Design review of the part built by this model. Coordinates are the model's own, in mm. A direction names the side the tool comes from. Give positions to 0.01 mm unless a question says otherwise; leave off trailing zeros. Order: outer loops, then holes, each group sorted by start corner. A loop starts at its lowest first (then second) coordinate and runs counter-clockwise, first axis right, second up. Notation, with made-up numbers: (-1.75, 81.25) -> (7.25, 81.25) arc R8 cw to (7.25, 87.25) -> close; hole circle Ø3 at (-8, 67). An arc over 180 degrees is marked (long way). Return JSON: item names as keys, results as strings.
```python
from build123d import *

# Parameters (mm, degrees)
BOSS_EXTRUDE1_DEPTH       = 13
SKETCH2_W                 = 26
SKETCH2_H                 = 9
CUT_EXTRUDE1_DEPTH        = 7
SKETCH3_W                 = 5.460158558
SKETCH3_H                 = 35.727642342
SKETCH3_W_2               = 6.990786849
SKETCH3_H_2               = 37.804269356
CUT_EXTRUDE2_DEPTH        = 56.362442143
M3X0_5_TAPPED_HOLE2_D     = 2.5
M3X0_5_TAPPED_HOLE2_DEPTH = 15
M3X0_5_TAPPED_HOLE2_TIP   = 0.751075774
M3X0_5_TAPPED_HOLE1_D     = 2.5
M3_CLEARANCE_HOLE1_D      = 3.4
CUT_EXTRUDE3_DEPTH        = 58.766772456
FILLET2_R                 = 3
CHAMFER1_SIZE             = 20
CHAMFER1_SIZE_2           = 3
CUT_EXTRUDE4_REACH        = 57.362
FILLET3_R                 = 2
CUT_EXTRUDE5_REACH        = 57.527
FILLET4_R                 = 2
M5X0_8_TAPPED_HOLE1_D     = 4.2
M5X0_8_TAPPED_HOLE1_DEPTH = 11.927025935
FILLET6_R                 = 5
CUT_EXTRUDE6_REACH        = 57.362
SKETCH19_W                = 7
SKETCH19_H                = 16
FILLET7_R                 = 1
CHAMFER2_SIZE             = 1.5
FILLET8_R                 = 0.5
FILLET9_R                 = 1


with BuildPart() as part:
    # Sketch1 → Boss-Extrude1 (new, symmetric)
    with BuildSketch(Plane.XY):
        Polygon((0, 0), (36, 0), (36, 36.17831254), (25.5, 40), (0, 17), align=None)
    extrude(amount=BOSS_EXTRUDE1_DEPTH, both=True)

    # Sketch2 → Cut-Extrude1 (cut)
    with BuildSketch(Plane.ZY):
        with Locations((0, 4.5)):
            Rectangle(SKETCH2_W, SKETCH2_H)
    extrude(amount=-CUT_EXTRUDE1_DEPTH, mode=Mode.SUBTRACT)

    # Sketch3 → Cut-Extrude2 (cut, through all)
    with BuildSketch(Plane.ZY):
        with Locations((10.730079279, 26.863821171)):
            Rectangle(SKETCH3_W, SKETCH3_H)
        with Locations((-11.495393425, 27.902134678)):
            Rectangle(SKETCH3_W_2, SKETCH3_H_2)
    extrude(amount=-CUT_EXTRUDE2_DEPTH, mode=Mode.SUBTRACT)

    # M3x0.5 Tapped Hole2
    with Locations(Plane(origin=(7, 5, -9.5), x_dir=(0, -1, 0), z_dir=(-1, 0, 0))):
        with Locations((0, 0), (0, 19)):
            Hole(M3X0_5_TAPPED_HOLE2_D / 2, depth=M3X0_5_TAPPED_HOLE2_DEPTH)
            with Locations((0, 0, -(M3X0_5_TAPPED_HOLE2_DEPTH + M3X0_5_TAPPED_HOLE2_TIP / 2))):  # 118° drill point
                Cone(0, M3X0_5_TAPPED_HOLE2_D / 2, M3X0_5_TAPPED_HOLE2_TIP, mode=Mode.SUBTRACT)

    # M3x0.5 Tapped Hole1 (through all)
    with Locations(Plane(origin=(3.5, 12.5, 8), x_dir=(1, 0, 0), z_dir=(0, 0, 1))):
        with Locations((0, 0)):
            Hole(M3X0_5_TAPPED_HOLE1_D / 2)

    # M3 Clearance Hole1 (through all)
    with Locations(Plane.XY.offset(13)):
        with Locations((27, 5)):
            Hole(M3_CLEARANCE_HOLE1_D / 2)

    # Sketch13 → Cut-Extrude3 (cut, through all)
    with BuildSketch(Plane.XY.offset(8)):
        Polygon((32, 18.871173631), (32, 26.992415753), (21.34884319, 30.869119792), (7, 17.927025935), (7, 11.927025935), (32, 11.927025935), align=None)
    extrude(amount=-CUT_EXTRUDE3_DEPTH, mode=Mode.SUBTRACT)

    # Fillet2
    fillet2_edges = [part.edges().sort_by_distance(p)[0] for p in [
        (7, 11.927025935, 0),
        (7, 17.927025935, 0),
        (21.34884319, 30.869119792, 0),
        (32, 26.992415753, 0),
        (32, 11.927025935, 0),
    ]]
    fillet(fillet2_edges, radius=FILLET2_R)

    # Chamfer1
    # the kernel refuses this chamfer: 20, 3 mm, written as the material it takes off along each edge
    with BuildSketch(Plane(origin=(84.844019059, 18.400543481, 8), x_dir=(-0.3420145720677014, -0.939677313880462, 0.005707737883485923), z_dir=(-0.9396926207859104, 0.3420201433256634, 0))) as chamfer1_piece_1:
        Polygon((CHAMFER1_SIZE * 0.999983710731, -CHAMFER1_SIZE * 0.00570773788349), (-CHAMFER1_SIZE_2 * 0.00570773788349, -CHAMFER1_SIZE_2 * 0.999983710731), (0, 0), align=None)
    extrude(amount=115.131305413, mode=Mode.SUBTRACT)
    with BuildSketch(Plane(origin=(84.844019059, 18.400543481, -8), x_dir=(0.08410022637244834, 0.23106347292932808, 0.9692970769593502), z_dir=(-0.9396926207859104, 0.3420201433256634, 0))) as chamfer1_piece_2:
        Polygon((CHAMFER1_SIZE_2 * 0.969297076959, -CHAMFER1_SIZE_2 * 0.245892611922), (-CHAMFER1_SIZE * 0.245892611922, -CHAMFER1_SIZE * 0.969297076959), (0, 0), align=None)
    extrude(amount=115.131305413, mode=Mode.SUBTRACT)

    # Sketch14 → Cut-Extrude4 (cut, up to next)
    with BuildSketch(Plane(origin=(36, 0, 0), x_dir=(0, 0, -1), z_dir=(1, 0, 0)), mode=Mode.PRIVATE) as cut_extrude4_sk1:
        Polygon((-3.405017352, 26), (3.405017352, 26), (5.096464069, 14), (-5.096464069, 14), align=None)
    cut_extrude4_tool1 = extrude(cut_extrude4_sk1.sketch, amount=-CUT_EXTRUDE4_REACH, mode=Mode.PRIVATE) & part.part
    add(cut_extrude4_tool1.solids().sort_by_distance((36, 19.602082, 0))[0], mode=Mode.SUBTRACT)

    # Fillet3
    fillet3_edges = [part.edges().sort_by_distance(p)[0] for p in [
        (33.926588844, 14, -5.096464069),
        (33.926588844, 14, 5.096464069),
        (33.893904368, 26, -3.405017352),
        (33.893904368, 26, 3.405017352),
    ]]
    fillet(fillet3_edges, radius=FILLET3_R)

    # Sketch16 → Cut-Extrude5 (cut, up to next)
    with BuildSketch(Plane(origin=(-8.45495018, 9.373966504, 0), x_dir=(0.7425697235686507, 0.669768770277607, 0), z_dir=(-0.669768770277607, 0.7425697235686507, 0)), mode=Mode.PRIVATE) as cut_extrude5_sk1:
        Polygon((19.386069095, 4.455184815), (19.386069095, -4.455184815), (34.386069095, -2.467646022), (34.386069095, 2.467646022), align=None)
    cut_extrude5_tool1 = extrude(cut_extrude5_sk1.sketch, amount=-CUT_EXTRUDE5_REACH, mode=Mode.PRIVATE) & part.part
    add(cut_extrude5_tool1.solids().sort_by_distance((10.976853, 26.900691, 0))[0], mode=Mode.SUBTRACT)

    # Fillet4
    fillet4_edges = [part.edges().sort_by_distance(p)[0] for p in [
        (7.280095329, 20.873010715, -4.455184815),
        (18.418641183, 30.919542269, -2.467646022),
        (18.418641183, 30.919542269, 2.467646022),
        (7.280095329, 20.873010715, 4.455184815),
    ]]
    fillet(fillet4_edges, radius=FILLET4_R)

    # M5x0.8 Tapped Hole1
    with Locations(Plane(origin=(0, 0, 0), x_dir=(-1, 0, 0), z_dir=(0, -1, 0))):
        with Locations((-17.5, 0)):
            Hole(M5X0_8_TAPPED_HOLE1_D / 2, depth=M5X0_8_TAPPED_HOLE1_DEPTH)

    # Fillet6
    fillet6_edges = [part.edges().sort_by_distance(p)[0] for p in [
        (36, 4.5, 13),
        (36, 4.5, -13),
    ]]
    fillet(fillet6_edges, radius=FILLET6_R)

    # Sketch19 → Cut-Extrude6 (cut, up to next)
    with BuildSketch(Plane.XZ, mode=Mode.PRIVATE) as cut_extrude6_sk1:
        with Locations((27.5, 0)):
            Rectangle(SKETCH19_W, SKETCH19_H)
    cut_extrude6_tool1 = extrude(cut_extrude6_sk1.sketch, amount=-CUT_EXTRUDE6_REACH, mode=Mode.PRIVATE) & part.part
    add(cut_extrude6_tool1.solids().sort_by_distance((27.5, 0, 0))[0], mode=Mode.SUBTRACT)

    # Fillet7
    fillet7_edges = [part.edges().sort_by_distance(p)[0] for p in [
        (24, 4.5, 8),
        (31, 4.5, -8),
        (24, 4.5, -8),
        (31, 4.5, 8),
    ]]
    fillet(fillet7_edges, radius=FILLET7_R)

    # Sketch21 → M5x0.8 Tapped Hole2 (revolve, cut)
    with BuildSketch(Plane(origin=(30.361844275, 38.2304334, 0), x_dir=(-0.9396926207859102, 0.3420201433256637, 0), z_dir=(0, 0, 1))):
        Polygon((0, 0), (0, 10), (2.675, 10), (2.1, 9.425), (2.1, 0), align=None)
    revolve(axis=Axis((32.533672185, 44.197481542, 0), (-0.3420201433256637, -0.9396926207859103, 0)), mode=Mode.SUBTRACT)

    # Chamfer2
    chamfer2_edges = [part.edges().sort_by_distance(p)[0] for p in [
        (3.5, 9, 8),
        (3.5, 9, -8),
    ]]
    chamfer(chamfer2_edges, length=CHAMFER2_SIZE)

    # Fillet8
    fillet8_edges = [part.edges().sort_by_distance(p)[0] for p in [
        (7, 9, 0),
    ]]
    fillet(fillet8_edges, radius=FILLET8_R)

    # Fillet9
    fillet9_edges = [part.edges().sort_by_distance(p)[0] for p in [
        (15.5, 9, 8),
        (15.5, 9, -8),
    ]]
    fillet(fillet9_edges, radius=FILLET9_R)


solid = part.part
```
Item 1: Add section A-A (y = 8). Give the boundary of the cut face in (x, z).
Result set:
{"outline": "(7, -13) -> (31, -13) arc R5 ccw to (36, -8) -> (36, 8) arc R5 ccw to (31, 13) -> (7, 13) -> close; hole circle Ø4.2 at (17.5, 0); hole (24, -7) arc R1 ccw to (25, -8) -> (30, -8) arc R1 ccw to (31, -7) -> (31, 7) arc R1 ccw to (30, 8) -> (25, 8) arc R1 ccw to (24, 7) -> close"}
Item 2: Wall thickness on L1, parallel to Z at x = 10.25, y = 5; L2, parallel to Z at x = 30, y = 5; L3, parallel to X at y = 7.5, z = -4.25: over which ranges is each line inside the solid? List them lowest first. Write a range as [from, to].
Result set:
{"L1": "z = [-13, -10.75], [-8.25, 8.25], [10.75, 13]", "L2": "z = [-13, -8], [8, 13]", "L3": "x = [7, 24], [31, 36]"}
Item 3: Add section B-B (x = 3.5). Give the boundary of the cut face in (y, z).
Result set:
{"outline": "(9, -6.5) -> (10.5, -8) -> (11.25, -8) -> (11.25, 8) -> (10.5, 8) -> (9, 6.5) -> close; (13.75, -8) -> (20.16, -8) -> (20.16, 8) -> (13.75, 8) -> close"}
Item 4: Mouldability with a two-part tool opening along Z and no side actions: class faces 1 (the face through (3.5, 9.7, -7.2)), 2 (the face through (3, 9, 0)), 3 (the face through (33.898, 14.706, 4.32)) as released by +Z, released by -Z, zero draft, split by the parting line, or undercut.
Result set:
{"face 1": "released by -Z", "face 2": "zero draft", "face 3": "undercut"}
Item 5: For pin 1 (1.5 mm diameter, centred on x = 8.5, z = 6.5, fed in from +Y); pin 2 (0.8 mm diameter, centred on y = 16, z = -1, fed in from +X); pin 3 (3 mm diameter, centred on x = 22, z = 11, fed in from +Y), all flat-tipped, find the tip position at first contact; note any pin that passes through.
Result set:
{"pin 1": "stops at y = 25.34", "pin 2": "stops at x = 7", "pin 3": "stops at y = 9"}
Item 6: Machinability: for faces 4 (the face through (21.467, 30.382, -0.094)), 5 (the face through (34.028, 20.335, -4.204)), 6 (the face through (3.5, 9.7, 7.2)), which of the approach directions +Z, -Z, +X, -X, +Y, -Y give a long, thin tool a straight path to every point of the face, cutting with its end or side? Answer none if there is none.
Result set:
{"face 4": "+Z, -Z", "face 5": "+X", "face 6": "+Z, -X, -Y"}
Item 7: Add section C-C (z = 0). Give the number of separate pieces and of enclosed holes in the cut face, plus the area to 3 significant figures.
Result set:
{"separate pieces": "5", "enclosed holes": "1", "area": "420 mm^2"}
